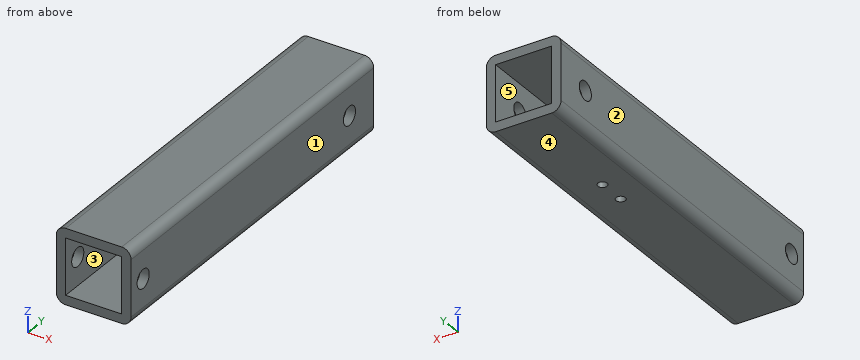
from build123d import *

# Parameters (mm, degrees)
F0_W     = 38.1
F0_H     = 38.1
F4_DEPTH = 254
F6_D     = 12.7
F6_DEPTH = 25.401
F1_D     = 12.7
F3_D     = 6.35
F3_DEPTH = 25.401


with BuildPart() as f4:
    # F0 (on Front) → F4 (new body)
    with BuildSketch(Plane.XZ):
        with BuildLine():
            Line((-19.05, -25.4), (19.05, -25.4))
            ThreePointArc((19.05, -25.4), (23.5401280605, -23.5401280605), (25.4, -19.05))
            Line((25.4, -19.05), (25.4, 19.05))
            ThreePointArc((25.4, 19.05), (23.5401280605, 23.5401280605), (19.05, 25.4))
            Line((19.05, 25.4), (-19.05, 25.4))
            ThreePointArc((-19.05, 25.4), (-23.5401280605, 23.5401280605), (-25.4, 19.05))
            Line((-25.4, 19.05), (-25.4, -19.05))
            ThreePointArc((-25.4, -19.05), (-23.5401280605, -23.5401280605), (-19.05, -25.4))
        make_face()
        Rectangle(F0_W, F0_H, mode=Mode.SUBTRACT)
    extrude(amount=-F4_DEPTH)

    # F6 (through all, one way)
    with BuildSketch(Plane(origin=(0, 0, 0), x_dir=(0, 1, 0), z_dir=(-1, 0, 0))):
        with Locations((12.7, 0), (228.6, 0)):
            Circle(F6_D / 2)
    extrude(amount=-F6_DEPTH, mode=Mode.SUBTRACT)

    # F1 (through all)
    with Locations(Plane.YZ):
        with Locations((12.7, 0), (228.6, 0)):
            Hole(F1_D / 2)

    # F3 (through all, one way)
    with BuildSketch(Plane.XY):
        with Locations((0, 171.45), (0, 152.4)):
            Circle(F3_D / 2)
    extrude(amount=-F3_DEPTH, mode=Mode.SUBTRACT)


solid = f4.part
Read the model definition and answer for the solid it produces. Units are mm, in the model's axes. Face numbers are marked on the shaded views. A direction names the side the tool comes from. Give positions to 0.01 mm unless a question says otherwise; leave off trailing zeros. Loops run counter-clockwise (first coordinate to the right, second up) from the corner with the lowest first, then second, coordinate; pieces in that order, holes last. Notation, with made-up numbers: (4, -14) -> (55, -14) arc R25 cw to (55, 15) -> close; hole circle Ø5 at (52, 18.25). An arc over 180 degrees is marked (long way). Use a Markdown table: item, result.
Q1. Section C-C, the plane x = -10 is taken. Determine the outline of the cut face in (y, z).
Solved:
| item | result |
|---|---|
| outline | (0, -25.4) -> (254, -25.4) -> (254, -19.05) -> (0, -19.05) -> close; (0, 19.05) -> (254, 19.05) -> (254, 25.4) -> (0, 25.4) -> close |
Q2. Each of these flat-tipped pins is pushed along its axis until it touches: pin 1 (5.5 mm diameter, centred on x = 0, y = 171.45, fed in from -Z); pin 2 (7.5 mm diameter, centred on x = 0, y = 152.4, fed in from -Z). Where does it stop, or does it pass through?
Solved:
| item | result |
|---|---|
| pin 1 | stops at z = 19.05 |
| pin 2 | stops at z = -25.4 |
Q3. Section D-D, the plane y = 171.45 is taken. Determine the outline of the cut face in (x, z) (3 decimals), then the cut area to 3 significant figures.
Solved:
| item | result |
|---|---|
| outline | (-25.4, -19.05) arc R6.35 ccw to (-19.05, -25.4) -> (-3.175, -25.4) -> (-3.175, -19.05) -> (-19.05, -19.05) -> (-19.05, 19.05) -> (19.05, 19.05) -> (19.05, -19.05) -> (3.175, -19.05) -> (3.175, -25.4) -> (19.05, -25.4) arc R6.35 ccw to (25.4, -19.05) -> (25.4, 19.05) arc R6.35 ccw to (19.05, 25.4) -> (-19.05, 25.4) arc R6.35 ccw to (-25.4, 19.05) -> close |
| area | 1,050 mm^2 |
Q4. Section B-B, the plane z = -11 is taken. Determine the outline of the cut face in (x, y).
Solved:
| item | result |
|---|---|
| outline | (-25.4, 0) -> (-19.05, 0) -> (-19.05, 254) -> (-25.4, 254) -> close; (19.05, 0) -> (25.4, 0) -> (25.4, 254) -> (19.05, 254) -> close |
Q5. Section A-A, the plane y = 228.6 is taken. Determine the outline of the cut face in (x, z).
Solved:
| item | result |
|---|---|
| outline | (-25.4, -19.05) arc R6.35 ccw to (-19.05, -25.4) -> (19.05, -25.4) arc R6.35 ccw to (25.4, -19.05) -> (25.4, -6.35) -> (19.05, -6.35) -> (19.05, -19.05) -> (-19.05, -19.05) -> (-19.05, -6.35) -> (-25.4, -6.35) -> close; (-25.4, 6.35) -> (-19.05, 6.35) -> (-19.05, 19.05) -> (19.05, 19.05) -> (19.05, 6.35) -> (25.4, 6.35) -> (25.4, 19.05) arc R6.35 ccw to (19.05, 25.4) -> (-19.05, 25.4) arc R6.35 ccw to (-25.4, 19.05) -> close |
Q6. Find the intervals of material crossed by line 1 along Y through (x, z) = (22.75, 0); line 2 along Z through (x, y) = (-4, 73.5), in increasing order.
Solved:
| item | result |
|---|---|
| line 1 | y = 0 to 6.35, 19.05 to 222.25, 234.95 to 254 |
| line 2 | z = -25.4 to -19.05, 19.05 to 25.4 |
Q7. A tool of negligible diameter and unlimited length cuts with its end or side. For the marked faces 4 and 5, from which of +Z, -Z, +X, -X, +Y, -Y can it reach the whole face along a straight path? Write none if from no direction.
Solved:
| item | result |
|---|---|
| face 4 | -Z, +X, -X, +Y, -Y |
| face 5 | +Y, -Y |
Q8. Determine the mould class of the marked faces 1, 2 and 3 for opening direction X: pulls with the +X half, pulls with the -X half, needs draft (parallel to the pull), parting line crosses it, or undercut.
Solved:
| item | result |
|---|---|
| face 1 | pulls with the +X half |
| face 2 | pulls with the -X half |
| face 3 | undercut |
